Verification items for the finished model (mm, model axes). A direction names the side the tool comes from. Round coordinates to 2 decimals unless told otherwise and drop trailing zeros. Order: outer loops, then holes, each group sorted by start corner. A loop starts at its lowest first (then second) coordinate and runs counter-clockwise, first axis right, second up. Notation, with made-up numbers: (56, 14.25) -> (89, 14.25) arc R16 ccw to (89, 20.25) -> close; hole circle Ø8 at (20.5, 53.25). An arc over 180 degrees is marked (long way). Return JSON: item names as keys, results as strings. Group by question number.
Item 1: Depth check by flat-ended pin: pin 1 Ø3 at (y, z) = (-11.5, 61.5) entering from -X; pin 2 Ø8 at (y, z) = (-23, 36) entering from -X; pin 3 Ø2.5 at (x, y) = (8.02, 8.02) entering from -Z; pin 4 Ø12 at (x, y) = (5.5, -7.5) entering from +Z. Enter the tip coordinate at first touch or a pass-through.
Item 2: Sectioned sample at A-A on x = 16.5. Record the cut outline in (y, z).
Item 3: Sectioned sample at B-B on z = 37.5. Record the cut outline in (x, y).
Item 4: Sectioned sample at C-C on z = 8.5. Give the number of separate pieces and of enclosed holes in the cut face, plus the area to 3 significant figures.
Item 5: Draft check along X on faces 3 (the cylindrical face through (-6.883, -30.995, 37.567)), 4 (the flat face through (0, 0, 12.7)), 5 (the flat face through (0, 0, 0)). Enter one of: pulls with the +X half, pulls with the -X half, needs draft (parallel to the pull), parting line crosses it, or undercut.
Item 6: Scan lines: probe 1 along X at (y, z) = (-4, 49); probe 2 along Y at (x, z) = (3.5, 44.5); probe 3 along Y at (x, z) = (-10.5, 31). Record each from-to range of solid material in increasing order. Write a range as from..to.
Item 7: Access from +Z, -Z, +X, -X, +Y, -Y to the whole of each face (thin tool, end or side, straight path). Record for faces 1 (the flat face through (14, -14, 76.2)), 2 (the cylindrical face through (-15.12, -11.59, 44.01)).
Item 8: Sectioned sample at D-D on y = 26.5. Record the cut outline in (x, z).
```python
from build123d import *

# Parameters (mm, degrees)
F0_R     = 31.75
F1_DEPTH = 76.2
F2_T     = -12.7
F3_R     = 0.79375
F4_DEPTH = 12.7


with BuildPart() as f1:
    # F0 (on Top) → F1 (new body)
    with BuildSketch(Plane.XY):
        Circle(F0_R)
    extrude(amount=F1_DEPTH)

    # F2
    f2_openings = [f1.faces().sort_by_distance(p)[0] for p in [
        (0, 0, 76.2),
    ]]
    offset(amount=F2_T, openings=f2_openings)

    # F3 (on face) → F4 (cut, through all)
    with BuildSketch(Plane.XY.offset(12.7)):
        with Locations((11.22532, -11.22532)):
            Circle(F3_R)
        with Locations((11.22532, -8.018086)):
            Circle(F3_R)
        with Locations((11.22532, -4.810851)):
            Circle(F3_R)
        with Locations((11.22532, -1.603617)):
            Circle(F3_R)
        with Locations((11.22532, 1.603617)):
            Circle(F3_R)
        with Locations((11.22532, 4.810851)):
            Circle(F3_R)
        with Locations((8.018086, 4.810851)):
            Circle(F3_R)
        with Locations((11.22532, 8.018086)):
            Circle(F3_R)
        with Locations((11.22532, 11.22532)):
            Circle(F3_R)
        with Locations((8.018086, 11.22532)):
            Circle(F3_R)
        with Locations((8.018086, 8.018086)):
            Circle(F3_R)
        with Locations((8.018086, 1.603617)):
            Circle(F3_R)
        with Locations((8.018086, -1.603617)):
            Circle(F3_R)
        with Locations((8.018086, -4.810851)):
            Circle(F3_R)
        with Locations((8.018086, -11.22532)):
            Circle(F3_R)
        with Locations((8.018086, -8.018086)):
            Circle(F3_R)
        with Locations((4.810851, -8.018086)):
            Circle(F3_R)
        with Locations((4.810851, -11.22532)):
            Circle(F3_R)
        with Locations((4.810851, -4.810851)):
            Circle(F3_R)
        with Locations((4.810851, -1.603617)):
            Circle(F3_R)
        with Locations((4.810851, 1.603617)):
            Circle(F3_R)
        with Locations((4.810851, 4.810851)):
            Circle(F3_R)
        with Locations((4.810851, 8.018086)):
            Circle(F3_R)
        with Locations((4.810851, 11.22532)):
            Circle(F3_R)
        with Locations((1.603617, -11.22532)):
            Circle(F3_R)
        with Locations((1.603617, -4.810851)):
            Circle(F3_R)
        with Locations((1.603617, -8.018086)):
            Circle(F3_R)
        with Locations((1.603617, -1.603617)):
            Circle(F3_R)
        with Locations((1.603617, 1.603617)):
            Circle(F3_R)
        with Locations((1.603617, 4.810851)):
            Circle(F3_R)
        with Locations((1.603617, 8.018086)):
            Circle(F3_R)
        with Locations((1.603617, 11.22532)):
            Circle(F3_R)
        with Locations((-1.603617, 11.22532)):
            Circle(F3_R)
        with Locations((-1.603617, -11.22532)):
            Circle(F3_R)
        with Locations((-4.810851, -11.22532)):
            Circle(F3_R)
        with Locations((-4.810851, -8.018086)):
            Circle(F3_R)
        with Locations((-1.603617, -8.018086)):
            Circle(F3_R)
        with Locations((-1.603617, -4.810851)):
            Circle(F3_R)
        with Locations((-4.810851, -4.810851)):
            Circle(F3_R)
        with Locations((-4.810851, -1.603617)):
            Circle(F3_R)
        with Locations((-1.603617, -1.603617)):
            Circle(F3_R)
        with Locations((-1.603617, 1.603617)):
            Circle(F3_R)
        with Locations((-4.810851, 1.603617)):
            Circle(F3_R)
        with Locations((-4.810851, 4.810851)):
            Circle(F3_R)
        with Locations((-1.603617, 4.810851)):
            Circle(F3_R)
        with Locations((-1.603617, 8.018086)):
            Circle(F3_R)
        with Locations((-4.810851, 8.018086)):
            Circle(F3_R)
        with Locations((-4.810851, 11.22532)):
            Circle(F3_R)
        with Locations((-8.018086, 8.018086)):
            Circle(F3_R)
        with Locations((-8.018086, 11.22532)):
            Circle(F3_R)
        with Locations((-11.22532, 11.22532)):
            Circle(F3_R)
        with Locations((-11.22532, 8.018086)):
            Circle(F3_R)
        with Locations((-11.22532, 4.810851)):
            Circle(F3_R)
        with Locations((-8.018086, 4.810851)):
            Circle(F3_R)
        with Locations((-11.22532, 1.603617)):
            Circle(F3_R)
        with Locations((-8.018086, 1.603617)):
            Circle(F3_R)
        with Locations((-8.018086, -1.603617)):
            Circle(F3_R)
        with Locations((-11.22532, -1.603617)):
            Circle(F3_R)
        with Locations((-11.22532, -4.810851)):
            Circle(F3_R)
        with Locations((-8.018086, -4.810851)):
            Circle(F3_R)
        with Locations((-8.018086, -8.018086)):
            Circle(F3_R)
        with Locations((-11.22532, -8.018086)):
            Circle(F3_R)
        with Locations((-11.22532, -11.22532)):
            Circle(F3_R)
        with Locations((-8.018086, -11.22532)):
            Circle(F3_R)
    extrude(amount=-F4_DEPTH, mode=Mode.SUBTRACT)


solid = f1.part
```
Recorded:
{
 "1": {"pin 1": "x = -30.13", "pin 2": "x = -25.44", "pin 3": "z = 0", "pin 4": "z = 12.7"},
 "2": {"outline": "(-27.13, 0) -> (27.13, 0) -> (27.13, 76.2) -> (9.52, 76.2) -> (9.52, 12.7) -> (-9.52, 12.7) -> (-9.52, 76.2) -> (-27.13, 76.2) -> close"},
 "3": {"outline": "circle Ø63.5 at (0, 0); hole circle Ø38.1 at (0, 0)"},
 "4": {"separate pieces": "1", "enclosed holes": "64", "area": "3,040 mm²"},
 "5": {"face 3": "parting line crosses it", "face 4": "undercut", "face 5": "needs draft"},
 "6": {"probe 1": "-31.5..-18.63, 18.63..31.5", "probe 2": "-31.56..-18.73, 18.73..31.56", "probe 3": "-29.96..-15.9, 15.9..29.96"},
 "7": {"face 1": "+Z, +X, -X, +Y, -Y", "face 2": "+Z"},
 "8": {"outline": "(-17.49, 0) -> (17.49, 0) -> (17.49, 76.2) -> (-17.49, 76.2) -> close"}
}
